Verification items for this drawing (mm, ordinates from the low corner). A direction names the side the tool comes from. Round coordinates to 2 decimals unless told otherwise and drop trailing zeros. Write each loop counter-clockwise with the first axis right and the second up, starting at its lowest first coordinate (ties: lowest second). Pieces come first, ordered by that corner, then holes. Notation, with made-up numbers: (34, -33.5) -> (44, -33.5) arc R19 ccw to (44, -15.5) -> close; hole circle Ø7 at (-2.5, 66.5). An arc over 180 degrees is marked (long way). One line per item, written item: value.
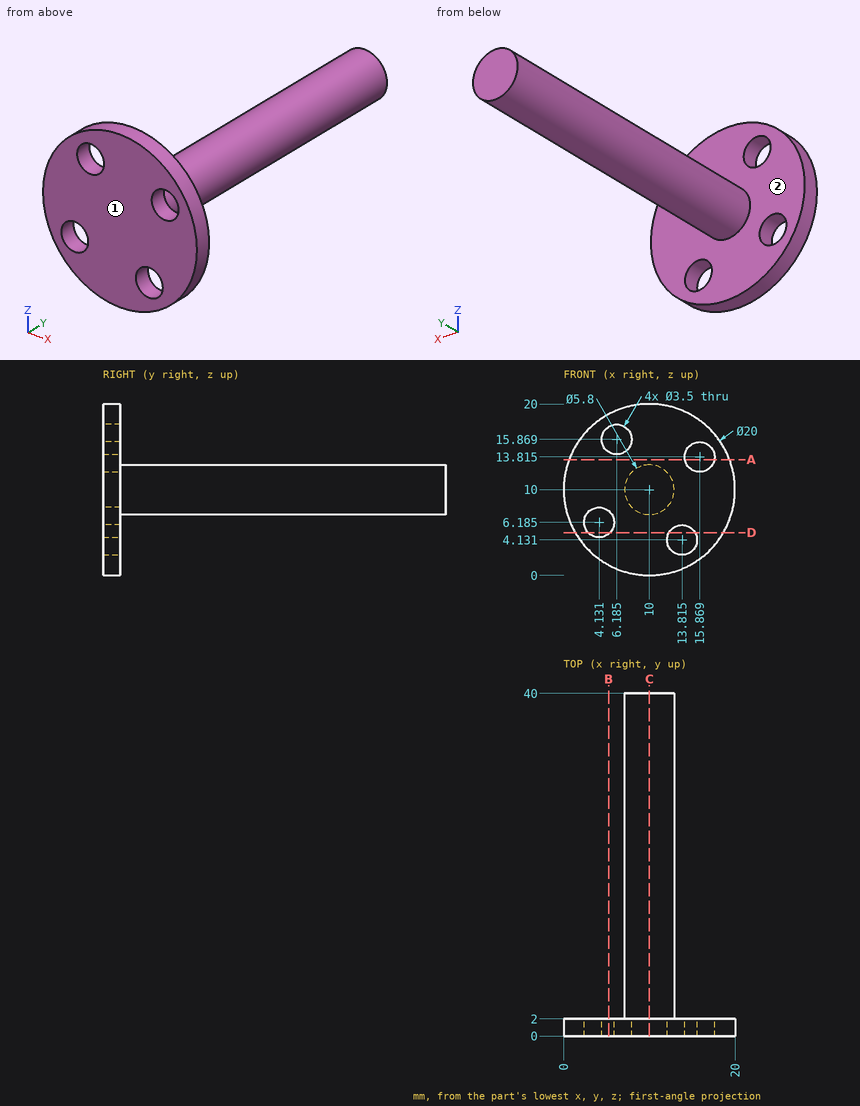
Item 1: Sectioned sample at A-A (z = 13.5). Enter the section's corners in (x, y).
Result set:
outline: (0.63, 0) -> (14.15, 0) -> (14.15, 2) -> (0.63, 2) -> close; (17.59, 0) -> (19.37, 0) -> (19.37, 2) -> (17.59, 2) -> close
Item 2: Tool access check on the marked faces 1 and 2. Record the directions out of +Z, -Z, +X, -X, +Y, -Y that give a thin tool (end or side, any length) a straight path to the whole face; none if there is none.
Result set:
face 1: +Z, -Z, +X, -X, -Y
face 2: +Y
Item 3: Sectioned sample at D-D (z = 5). Enter the section's corners in (x, y) (1 decimal).
Result set:
outline: (1.3, 0) -> (2.8, 0) -> (2.8, 2) -> (1.3, 2) -> close; (5.4, 0) -> (12.3, 0) -> (12.3, 2) -> (5.4, 2) -> close; (15.3, 0) -> (18.7, 0) -> (18.7, 2) -> (15.3, 2) -> close
Item 4: Depth check by flat-ended pin: pin 1 (4.5 mm diameter, centred on x = 15.87, z = 13.81, fed in from +Y); pin 2 (4 mm diameter, centred on x = 9, y = 14.5, fed in from -Z); pin 3 (8 mm diameter, centred on x = 4, y = 35, fed in from -Z). Enter the tip coordinate at first touch or a pass-through.
Result set:
pin 1: y = 2
pin 2: z = 7.1
pin 3: z = 7.9
Item 5: Sectioned sample at B-B (x = 5.25). Enter the section's corners in (y, z).
Result set:
outline: (0, 1.2) -> (2, 1.2) -> (2, 4.84) -> (0, 4.84) -> close; (0, 7.53) -> (2, 7.53) -> (2, 14.39) -> (0, 14.39) -> close; (0, 17.35) -> (2, 17.35) -> (2, 18.8) -> (0, 18.8) -> close
Item 6: Sectioned sample at C-C (x = 10). Enter the section's corners in (y, z).
Result set:
outline: (0, 0) -> (2, 0) -> (2, 7.1) -> (40, 7.1) -> (40, 12.9) -> (2, 12.9) -> (2, 20) -> (0, 20) -> close
Item 7: Material ranges on line 1 along Y through (x, z) = (7, 8.5); line 2 along X through (y, z) = (3, 9.5), recorded low to high.
Result set:
line 1: 0 to 2
line 2: 7.14 to 12.86
